CAD build for the part. Positions are in the model's coordinates, mm. Face numbers are marked on the shaded views. A direction names the side the tool comes from. Coordinates: 2 decimals unless noted, no trailing zeros. Loops run counter-clockwise (first coordinate to the right, second up) from the corner with the lowest first, then second, coordinate; pieces in that order, holes last. Notation, with made-up numbers: (5, -16.5) -> (40, -16.5) arc R15 ccw to (40, -3.5) -> close; hole circle Ø2 at (7, -38). An arc over 180 degrees is marked (long way). Write each question's results on one line, items separated by ' | '.
from build123d import *

# Parameters (mm, degrees)
F0_R     = 8.5
F1_DEPTH = 3
F2_DEPTH = 13


with BuildPart() as f1:
    # F0 (on Top) → F1 (new body)
    with BuildSketch(Plane.XY):
        Polygon((-23.094011, 20), (-11.547005, 20), (-5.773503, 30), align=None)
        Polygon((5.773503, 30), (11.547005, 20), (23.094011, 20), align=None)
        Polygon((11.547005, 20), (5.773503, 10), (11.547005, 0), (23.094011, 0), (28.867513, 10), (23.094011, 20), align=None)
        with Locations((17.320508, 10)):
            Circle(F0_R, mode=Mode.SUBTRACT)
        Polygon((-5.773503, -30), (-11.547005, -20), (-23.094011, -20), align=None)
        Polygon((23.094011, 0), (11.547005, 0), (5.773503, -10), (11.547005, -20), (23.094011, -20), (28.867513, -10), align=None)
        with Locations((17.320508, -10)):
            Circle(F0_R, mode=Mode.SUBTRACT)
        Polygon((28.867513, 10), (23.094011, 0), (28.867513, -10), align=None)
        Polygon((-28.867513, -10), (-23.094011, 0), (-28.867513, 10), align=None)
        Polygon((-11.547005, 20), (-5.773503, 10), (5.773503, 10), (11.547005, 20), (5.773503, 30), (-5.773503, 30), align=None)
        with Locations((0, 20)):
            Circle(F0_R, mode=Mode.SUBTRACT)
        Polygon((5.773503, 10), (-5.773503, 10), (-11.547005, 0), (-5.773503, -10), (5.773503, -10), (11.547005, 0), align=None)
        Circle(F0_R, mode=Mode.SUBTRACT)
        Polygon((5.773503, -10), (-5.773503, -10), (-11.547005, -20), (-5.773503, -30), (5.773503, -30), (11.547005, -20), align=None)
        with Locations((0, -20)):
            Circle(F0_R, mode=Mode.SUBTRACT)
        Polygon((23.094011, -20), (11.547005, -20), (5.773503, -30), align=None)
        Polygon((-5.773503, -10), (-11.547005, 0), (-23.094011, 0), (-28.867513, -10), (-23.094011, -20), (-11.547005, -20), align=None)
        with Locations((-17.320508, -10)):
            Circle(F0_R, mode=Mode.SUBTRACT)
        Polygon((-11.547005, 0), (-5.773503, 10), (-11.547005, 20), (-23.094011, 20), (-28.867513, 10), (-23.094011, 0), align=None)
        with Locations((-17.320508, 10)):
            Circle(F0_R, mode=Mode.SUBTRACT)
        with Locations((0, 20)):
            Circle(F0_R)
        with Locations((17.320508, 10)):
            Circle(F0_R)
        Circle(F0_R)
        with Locations((17.320508, -10)):
            Circle(F0_R)
        with Locations((0, -20)):
            Circle(F0_R)
        with Locations((-17.320508, -10)):
            Circle(F0_R)
        with Locations((-17.320508, 10)):
            Circle(F0_R)
    extrude(amount=F1_DEPTH)

    # F0 (on Top) → F2 (join)
    with BuildSketch(Plane.XY):
        Polygon((5.773503, 10), (-5.773503, 10), (-11.547005, 0), (-5.773503, -10), (5.773503, -10), (11.547005, 0), align=None)
        Circle(F0_R, mode=Mode.SUBTRACT)
        Polygon((-5.773503, -10), (-11.547005, 0), (-23.094011, 0), (-28.867513, -10), (-23.094011, -20), (-11.547005, -20), align=None)
        with Locations((-17.320508, -10)):
            Circle(F0_R, mode=Mode.SUBTRACT)
        Polygon((-11.547005, 20), (-5.773503, 10), (5.773503, 10), (11.547005, 20), (5.773503, 30), (-5.773503, 30), align=None)
        with Locations((0, 20)):
            Circle(F0_R, mode=Mode.SUBTRACT)
        Polygon((5.773503, -10), (-5.773503, -10), (-11.547005, -20), (-5.773503, -30), (5.773503, -30), (11.547005, -20), align=None)
        with Locations((0, -20)):
            Circle(F0_R, mode=Mode.SUBTRACT)
        Polygon((23.094011, 0), (11.547005, 0), (5.773503, -10), (11.547005, -20), (23.094011, -20), (28.867513, -10), align=None)
        with Locations((17.320508, -10)):
            Circle(F0_R, mode=Mode.SUBTRACT)
        Polygon((11.547005, 20), (5.773503, 10), (11.547005, 0), (23.094011, 0), (28.867513, 10), (23.094011, 20), align=None)
        with Locations((17.320508, 10)):
            Circle(F0_R, mode=Mode.SUBTRACT)
        Polygon((-11.547005, 0), (-5.773503, 10), (-11.547005, 20), (-23.094011, 20), (-28.867513, 10), (-23.094011, 0), align=None)
        with Locations((-17.320508, 10)):
            Circle(F0_R, mode=Mode.SUBTRACT)
    extrude(amount=F2_DEPTH)


solid = f1.part
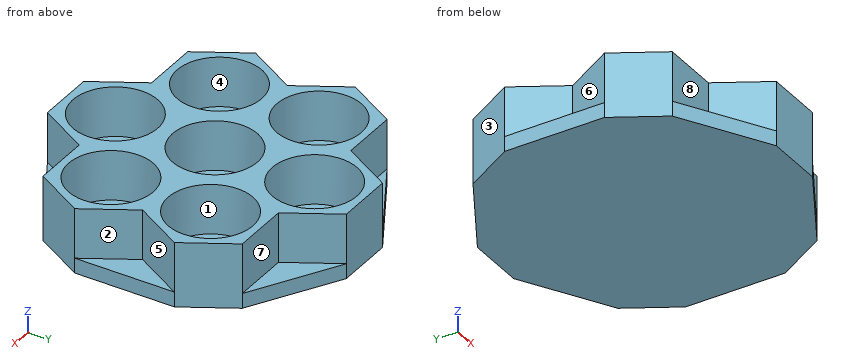
1) Slice it at B-B (x = 0). Write the cut outline in (y, z).
Outcome:
outline: (-30, 0) -> (30, 0) -> (30, 13) -> (28.5, 13) -> (28.5, 3) -> (11.5, 3) -> (11.5, 13) -> (8.5, 13) -> (8.5, 3) -> (-8.5, 3) -> (-8.5, 13) -> (-11.5, 13) -> (-11.5, 3) -> (-28.5, 3) -> (-28.5, 13) -> (-30, 13) -> close
2) Slice it at A-A (z = 4). Write the cut outline in (x, y).
Outcome:
outline: (-28.87, -10) -> (-23.09, -20) -> (-11.55, -20) -> (-5.77, -30) -> (5.77, -30) -> (11.55, -20) -> (23.09, -20) -> (28.87, -10) -> (23.09, 0) -> (28.87, 10) -> (23.09, 20) -> (11.55, 20) -> (5.77, 30) -> (-5.77, 30) -> (-11.55, 20) -> (-23.09, 20) -> (-28.87, 10) -> (-23.09, 0) -> close; hole circle Ø17 at (-17.32, -10); hole circle Ø17 at (-17.32, 10); hole circle Ø17 at (0, -20); hole circle Ø17 at (0, 0); hole circle Ø17 at (0, 20); hole circle Ø17 at (17.32, -10); hole circle Ø17 at (17.32, 10)
3) Slice it at C-C (y = 3). Write the cut outline in (x, z).
Outcome:
outline: (-28.87, 0) -> (28.87, 0) -> (28.87, 3) -> (24.83, 3) -> (24.83, 13) -> (22.14, 13) -> (22.14, 3) -> (12.5, 3) -> (12.5, 13) -> (7.95, 13) -> (7.95, 3) -> (-7.95, 3) -> (-7.95, 13) -> (-12.5, 13) -> (-12.5, 3) -> (-22.14, 3) -> (-22.14, 13) -> (-24.83, 13) -> (-24.83, 3) -> (-28.87, 3) -> close
4) Drill centre lines: L1, parallel to Y at x = 17, z = 8.5; L2, parallel to X at y = 10, z = 9.5; L3, parallel to X at y = -4, z = 3.5. Where is each one in solid material? Low to high. Write a range as from..to.
Outcome:
L1: y = -20..-18.49, -1.51..1.51, 18.49..20 | L2: x = -28.87..-25.82, -8.82..8.82, 25.82..28.87 | L3: x = -25.4..-23.34, -11.3..-7.5, 7.5..11.3, 23.34..25.4
5) Which spindle directions (+Z, -Z, +X, -X, +Y, -Y) get a long thin tool onto all of the face, cutting with end or side? Do the marked faces 5, 6, 7 and 8. Say none if no direction does.
Outcome:
face 5: +Z, +X | face 6: +Z, -X | face 7: +Z, +X, +Y | face 8: +Z, -X, -Y
6) Two-plate mould, pull along X, no slides. Class the marked faces 1, 2, 3 and 4: pulls with the +X half, pulls with the -X half, needs draft (parallel to the pull), parting line crosses it, or undercut.
Outcome:
face 1: undercut | face 2: pulls with the +X half | face 3: pulls with the -X half | face 4: undercut
7) Slice it at D-D (x = -7). Write the cut outline in (y, z).
Outcome:
outline: (-29.29, 0) -> (29.29, 0) -> (29.29, 3) -> (27.88, 3) -> (27.88, 13) -> (24.82, 13) -> (24.82, 3) -> (15.18, 3) -> (15.18, 13) -> (4.82, 13) -> (4.82, 3) -> (-4.82, 3) -> (-4.82, 13) -> (-15.18, 13) -> (-15.18, 3) -> (-24.82, 3) -> (-24.82, 13) -> (-27.88, 13) -> (-27.88, 3) -> (-29.29, 3) -> close
8) Pin check, flat tips, straight feed: pin 1 (2 mm diameter, centred on x = 15.5, z = 1.5, fed in from -Y); pin 2 (1 mm diameter, centred on x = 6.5, y = -2, fed in from +Z); pin 3 (5 mm diameter, centred on x = -16.5, z = 8, fed in from +Y). Stop position of each tip, or through.
Outcome:
pin 1: stops at y = -24.96 | pin 2: stops at z = 3 | pin 3: stops at y = 20
